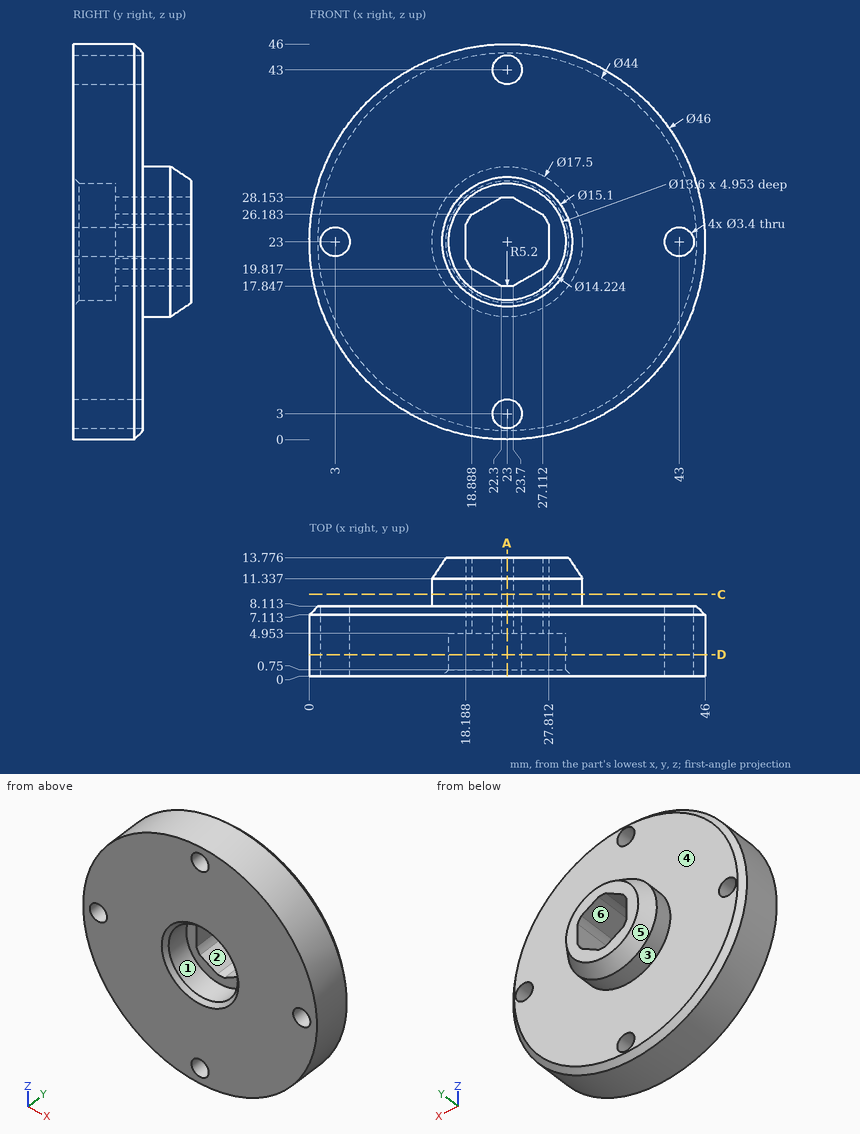
Source: three-view drawing plus pictorial views. Frame: mm from the lowest corner of the part. A direction names the side the tool comes from. Give positions to 0.01 mm unless a question says otherwise; leave off trailing zeros. Order: outer loops, then holes, each group sorted by start corner. A loop starts at its lowest first (then second) coordinate and runs counter-clockwise, first axis right, second up. Notation, with made-up numbers: M 36,-9 L 73,-9 A13 ccw 73,-2 Z; hole C 48,57 d8. An arc over 180 degrees is marked long. Return JSON: item names as keys, results as strings.
1) Section query D-D on y = 2.5. Output: boundary loops of the cut face in (x, z), and give its area (3 significant figures).
Taken from the geometry:
{"outline": "C 23,23 d46; hole C 3,23 d3.4; hole C 23,23 d13.6; hole C 23,3 d3.4; hole C 23,43 d3.4; hole C 43,23 d3.4", "area": "1,480 mm2"}
2) Contact query for flat-ended pins moving along their axis: pin 1 (4 mm diameter, centred on y = 3.5, z = 32.5, fed in from +X); pin 2 (1 mm diameter, centred on x = 11, y = 6, fed in from +Z); pin 3 (4.5 mm diameter, centred on y = 9.5, z = 22.5, fed in from -X). Output: stop coordinate, or through.
Taken from the geometry:
{"pin 1": "stops at x = 44.74", "pin 2": "stops at z = 42.92", "pin 3": "stops at x = 0.14"}
3) Section query A-A on x = 23. Count the separate pieces of the cut face and the enclosed holes in it.
Taken from the geometry:
{"separate pieces": "4", "enclosed holes": "0"}
4) Section query C-C on y = 9.5. Output: boundary loops of the cut face in (x, z).
Taken from the geometry:
{"outline": "C 23,23 d17.5; hole M 18.19,21.03 A5.2 ccw 18.89,19.82 L 22.3,17.85 A5.2 ccw 23.7,17.85 L 27.11,19.82 A5.2 ccw 27.81,21.03 L 27.81,24.97 A5.2 ccw 27.11,26.18 L 23.7,28.15 A5.2 ccw 22.3,28.15 L 18.89,26.18 A5.2 ccw 18.19,24.97 Z"}
5) Line query: L1, parallel to Y at x = 33.5, z = 8; L2, parallel to Z at x = 43, y = 2.25 (1 decimal). Output: solid intervals per line, ascending. Write a range as [from, to].
Taken from the geometry:
{"L1": "y = [0, 8.11]", "L2": "z = [11.6, 21.3], [24.7, 34.4]"}
6) Access query for the marked faces 5 and 6. Directions: +Z, -Z, +X, -X, +Y, -Y. A direction counts if a zero-diameter tool reaches every point of the face in a straight line with its end or side. Return the directions, or none.
Taken from the geometry:
{"face 5": "+Y", "face 6": "+Y, -Y"}
7) Mould query, pull axis Z, two halves, no side actions, for the marked faces 1, 2, 3 and 4. Classes: released by +Z, released by -Z, zero draft, split by the parting line, or undercut.
Taken from the geometry:
{"face 1": "undercut", "face 2": "undercut", "face 3": "split by the parting line", "face 4": "zero draft"}
